from build123d import *

# Parameters (mm, degrees)
BOSS_EXTRUDE1_DEPTH = 30
BOSS_EXTRUDE2_START = -30
BOSS_EXTRUDE2_DEPTH = 30
SKETCH4_R           = 25
CUT_EXTRUDE2_DEPTH  = 30
BOSS_EXTRUDE3_DEPTH = 2
BOSS_EXTRUDE4_START = -10
BOSS_EXTRUDE4_DEPTH = 10
SKETCH7_R           = 23
CUT_EXTRUDE4_DEPTH  = 27


with BuildPart() as part:
    # Sketch2 → Boss-Extrude1 (new body)
    with BuildSketch(Plane.XY):
        with BuildLine():
            Line((3, 0), (5, 0))
            ThreePointArc((5, 0), (18, 13), (31, 0))
            Line((31, 0), (33, 0))
            ThreePointArc((33, 0), (18, 15), (3, 0))
        make_face()
    extrude(amount=BOSS_EXTRUDE1_DEPTH)

    # Sketch3 → Boss-Extrude2 (add)
    with BuildSketch(Plane.XY.offset(BOSS_EXTRUDE2_START)):
        with BuildLine():
            Line((3, 0), (5, 0))
            ThreePointArc((5, 0), (18, 13), (31, 0))
            Line((31, 0), (33, 0))
            ThreePointArc((33, 0), (18, 15), (3, 0))
        make_face()
    extrude(amount=BOSS_EXTRUDE2_DEPTH)

    # Sketch4 → Cut-Extrude2 (cut)
    with BuildSketch(Plane(origin=(0, 0, 0), x_dir=(1, 0, 0), z_dir=(0, 1, 0))):
        with Locations((18, 25)):
            Circle(SKETCH4_R)
    extrude(amount=CUT_EXTRUDE2_DEPTH, mode=Mode.SUBTRACT)

    # Sketch5 → Boss-Extrude3 (add)
    with BuildSketch(Plane.XY.offset(30)):
        with BuildLine():
            Line((4, 0), (5, 0))
            ThreePointArc((5, 0), (18, 13), (31, 0))
            Line((31, 0), (32, 0))
            ThreePointArc((32, 0), (18, 14), (4, 0))
        make_face()
    extrude(amount=BOSS_EXTRUDE3_DEPTH)

    # Sketch6 → Boss-Extrude4 (add)
    with BuildSketch(Plane.XY.offset(BOSS_EXTRUDE4_START)):
        with BuildLine():
            Line((5, 0), (4, 0))
            ThreePointArc((4, 0), (18, 14), (32, 0))
            Line((32, 0), (31, 0))
            ThreePointArc((31, 0), (18, 13), (5, 0))
        make_face()
    extrude(amount=BOSS_EXTRUDE4_DEPTH)

    # Sketch7 → Cut-Extrude4 (cut)
    with BuildSketch(Plane(origin=(0, 0, 0), x_dir=(1, 0, 0), z_dir=(0, 1, 0))):
        with Locations((18, 25)):
            Circle(SKETCH7_R)
    extrude(amount=CUT_EXTRUDE4_DEPTH, mode=Mode.SUBTRACT)


solid = part.part
Model file for the job. Use its own axes, mm. A direction names the side the tool comes from. Coordinates: 2 decimals unless noted, no trailing zeros. Order: outer loops, then holes, each group sorted by start corner. A loop starts at its lowest first (then second) coordinate and runs counter-clockwise, first axis right, second up. Notation, with made-up numbers: M 83,50.25 L 91,50.25 A20 cw 91,67.25 Z; hole C -33.5,76.5 d4. An arc over 180 degrees is marked long. Return JSON: item names as keys, results as strings.
1. Saw through at D-D (y = 9). Give the cut face in (x, z).
Ans:
{"outline": "M 6,-3.07 A25 cw 7.28,-2.42 L 7.28,-4.65 A23 cw 8.62,-4 L 8.62,32 L 7.28,32 L 7.28,30 L 6,30 Z; M 27.38,-4 A23 cw 28.72,-4.65 L 28.72,-2.42 A25 cw 30,-3.07 L 30,30 L 28.72,30 L 28.72,32 L 27.38,32 Z"}
2. Saw through at C-C (z = 4.5). Give the cut face in (x, y), and give its area (3 significant figures).
Ans:
{"outline": "M 3,0 L 5,0 A13 cw 31,0 L 33,0 A15 ccw Z", "area": "88.0 mm^2"}
3. Saw through at B-B (x = 18). Give the cut face in (y, z).
Ans:
{"outline": "M 13,-2 L 14,-2 L 14,0 L 15,0 L 15,30 L 14,30 L 14,32 L 13,32 Z"}
4. Saw through at A-A (y = 4.5). Give the cut face in (x, z).
Ans:
{"outline": "M 3.69,-4.5 A25 cw 4.74,-3.8 L 4.74,-6.21 A23 cw 5.8,-5.5 L 5.8,32 L 4.74,32 L 4.74,30 L 3.69,30 Z; M 30.2,-5.5 A23 cw 31.26,-6.21 L 31.26,-3.8 A25 cw 32.31,-4.5 L 32.31,30 L 31.26,30 L 31.26,32 L 30.2,32 Z"}
5. Drill centre lines: probe 1 along X at (y, z) = (1, 19); probe 2 along X at (y, z) = (7.5, -2); probe 3 along Y at (x, z) = (18, 25.5). Where is each one in solid material? Low to high.
Ans:
{"probe 1": "3.03 to 5.04, 30.96 to 32.97", "probe 2": "5.01 to 7.38, 28.62 to 30.99", "probe 3": "13 to 15"}
6. Flat gauge pins, fed straight in: pin 1 (1 mm diameter, centred on y = 7.5, z = 13.5, fed in from +X); pin 2 (6 mm diameter, centred on x = 6.5, y = 9, fed in from -Z); pin 3 (1 mm diameter, centred on x = 19, z = 27.5, fed in from +Y). Where does each tip first touch, or does it go through?
Ans:
{"pin 1": "x = 31.27", "pin 2": "z = -5.73", "pin 3": "y = 14.99"}
7. Pull direction X, two halves, no side cores. Call faces 1 (the face through (18, 15, 12)), 2 (the face through (32, 0, 12)), 3 (the face through (17.9, 14, -1.6)), 4 (the face through (17.9, 13.2, -2)): +X half, -X half, draft (parallel to the pull), parting line (faces both ways), or undercut.
Ans:
{"face 1": "parting line", "face 2": "draft", "face 3": "undercut", "face 4": "undercut"}
8. Tool access for faces 5 (the face through (17.9, 14.2, 30)), 6 (the face through (4, 0, 12)): list every direction of +Z, -Z, +X, -X, +Y, -Y with a clear straight run to the whole face (end or side of a thin tool).
Ans:
{"face 5": "+Z, +Y", "face 6": "+Z, -Z, +X, -X, -Y"}
